The model under review builds one solid part; all positions refer to its coordinate system, in mm. A direction names the side the tool comes from. Coordinates: 2 decimals unless noted, no trailing zeros. Write each loop counter-clockwise with the first axis right and the second up, starting at its lowest first coordinate (ties: lowest second). Pieces come first, ordered by that corner, then holes. Notation, with made-up numbers: (-36.75, 44) -> (-18.75, 44) arc R17 ccw to (-18.75, 57) -> close; hole circle Ø11 at (-33.5, 40.25). An arc over 180 degrees is marked (long way). Put each result on its own line as item: value. Start each with the question number.
from build123d import *

# Parameters (mm, degrees)
BOSS_EXTRUDE1_DEPTH = 2
SKETCH2_W           = 1.82062343
SKETCH2_H           = 2
BOSS_EXTRUDE2_DEPTH = 3
BOSS_EXTRUDE3_DEPTH = 3


with BuildPart() as part:
    # Sketch1 → Boss-Extrude1 (new body)
    with BuildSketch(Plane.XY):
        Polygon((0, 0), (6, 0), (6, 2), (4, 2), (1, 5), (0, 5), align=None)
    extrude(amount=-BOSS_EXTRUDE1_DEPTH)



with BuildPart() as body_2:
    # Sketch2 → Boss-Extrude2 (new body)
    with BuildSketch(Plane.ZY):
        with Locations((0.910311715, 4)):
            Rectangle(SKETCH2_W, SKETCH2_H)
    extrude(amount=-BOSS_EXTRUDE2_DEPTH)


with BuildPart() as part_1:
    add(part.part)

    add(body_2.part)  # Boss-Extrude3 merges body 2
    # Sketch3 → Boss-Extrude3 (add)
    with BuildSketch(Plane.XZ.offset(-3)):
        Polygon((0, 0), (3, 0), (0, 1.82062343), align=None)
    extrude(amount=BOSS_EXTRUDE3_DEPTH)


solid = part_1.part
1. Wall thickness on line 1 (Y direction, x = 1.8, z = 0.9); line 2 (X direction, y = 3.2, z = 0.15); line 3 (Y direction, x = 4.3, z = -0.3): over which ranges is each line inside the solid? List them lowest first. Write a range as from..to.
2. Consider section C-C on z = -0.2. State the section outline as (x, y) points, then the cut area to 3 significant figures.
3. Tool access review of faces 1 (the flat face through (1.1, 5, 0.3)), 2 (the flat face through (4, 1, 0)), 3 (the flat face through (2, 3, 1)), 4 (the flat face through (3, 3, -1)), 5 (the flat face through (5, 2, -1)): name each direction out of +Z, -Z, +X, -X, +Y, -Y from which nothing blocks a thin tool from reaching the whole face with its end or side.
4. Consider section B-B on x = 1.3. State the section outline as (y, z) points.
5. Insertion check: P1, Ø0.5, axis at y = 4.5, z = 1, coming from the +X side; P2, Ø1.5, axis at x = 4, y = 1.5, coming from the +Z side. Each pin has a flat end and moves straight along its axis. Give the tip position at first contact, or say it passes through.
6. Consider section A-A on y = 3.65. State the section outline as (x, z) points, then the cut area to 3 significant figures.
7. Consider section D-D on y = 2.9. State the section outline as (x, z) points.
Output values:
1. line 1: y = 3..5
1. line 2: x = 0..3
1. line 3: y = 0..2
2. outline: (0, 0) -> (6, 0) -> (6, 2) -> (4, 2) -> (1, 5) -> (0, 5) -> close
2. area: 19.5 mm^2
3. face 1: +Z, -Z, +X, -X, +Y
3. face 2: +Z, +X, +Y, -Y
3. face 3: +Z, +X, -Y
3. face 4: -Z, +X, +Y
3. face 5: +Z, -Z, +X, +Y
4. outline: (0, -2) -> (4.7, -2) -> (4.7, 0) -> (5, 0) -> (5, 1.82) -> (3, 1.82) -> (3, 1.03) -> (0, 1.03) -> close
5. P1: stops at x = 3
5. P2: stops at z = 0
6. outline: (0, -2) -> (2.35, -2) -> (2.35, 0) -> (3, 0) -> (3, 1.82) -> (0, 1.82) -> close
6. area: 10.2 mm^2
7. outline: (0, -2) -> (3.1, -2) -> (3.1, 0) -> (3, 0) -> (0, 1.82) -> close
